Verification items for the finished model (mm, model axes). Face numbers are marked on the shaded views. A direction names the side the tool comes from. Give positions to 0.01 mm unless a question says otherwise; leave off trailing zeros. Write each loop counter-clockwise with the first axis right and the second up, starting at its lowest first coordinate (ties: lowest second). Pieces come first, ordered by that corner, then holes. Notation, with made-up numbers: M 65.25,40.25 L 100.25,40.25 A12 cw 100.25,45.25 Z; hole C 50,12.25 d3. An arc over 180 degrees is marked long. Answer as a JSON object with one key per item and string values.
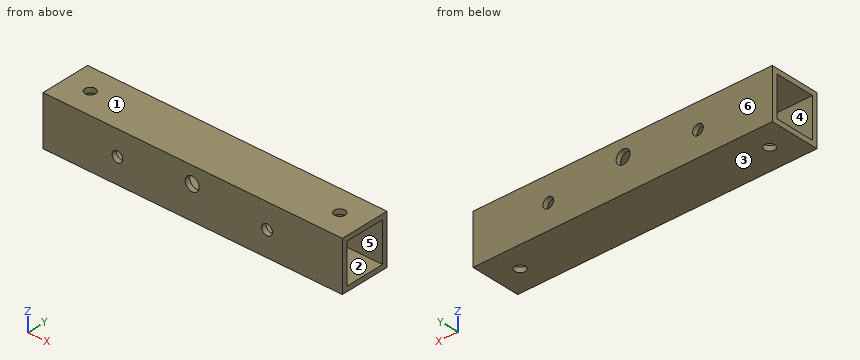
```python
from build123d import *

# Parameters (mm, degrees)
SKETCH_1_W          = 15
SKETCH_1_H          = 15
SKETCH_1_W_2        = 12
SKETCH_1_H_2        = 12
EXTRUDE_1_DEPTH     = 90
SKETCH_2_R          = 2.1
SKETCH_2_R_2        = 1.6
CUT_EXTRUDE_1_DEPTH = 92.549167118
SKETCH_3_R          = 1.6
CUT_EXTRUDE_2_DEPTH = 92.549167118


with BuildPart() as part:
    # ｽｹｯﾁ1 → ﾎﾞｽ - 押し出し1 (new body)
    with BuildSketch(Plane(origin=(0, 0, 0), x_dir=(0, 0, -1), z_dir=(1, 0, 0))):
        Rectangle(SKETCH_1_W, SKETCH_1_H)
        Rectangle(SKETCH_1_W_2, SKETCH_1_H_2, mode=Mode.SUBTRACT)
    extrude(amount=EXTRUDE_1_DEPTH)

    # ｽｹｯﾁ2 → ｶｯﾄ - 押し出し1 (cut, through all)
    with BuildSketch(Plane(origin=(0, 7.5, 0), x_dir=(1, 0, 0), z_dir=(0, 1, 0))):
        with Locations(Location((44.860461956, -2.501947466, 0), (0, 0, 270))):
            Circle(SKETCH_2_R)
        with Locations(Location((22.360461956, 0, 0), (0, 0, 270))):
            Circle(SKETCH_2_R_2)
        with Locations(Location((67.360461956, 0, 0), (0, 0, 270))):
            Circle(SKETCH_2_R_2)
    extrude(amount=-CUT_EXTRUDE_1_DEPTH, mode=Mode.SUBTRACT)

    # ｽｹｯﾁ3 → ｶｯﾄ - 押し出し2 (cut, through all)
    with BuildSketch(Plane.XY.offset(7.5)):
        with Locations((7.5, 0)):
            Circle(SKETCH_3_R)
        with Locations((82.5, 0)):
            Circle(SKETCH_3_R)
    extrude(amount=-CUT_EXTRUDE_2_DEPTH, mode=Mode.SUBTRACT)


solid = part.part
```
1) Section check C-C on x = 82.5. Record the boundary of the cut face in (y, z).
Completed:
{"outline": "M -7.5,-7.5 L -1.6,-7.5 L -1.6,-6 L -6,-6 L -6,6 L -1.6,6 L -1.6,7.5 L -7.5,7.5 Z; M 1.6,-7.5 L 7.5,-7.5 L 7.5,7.5 L 1.6,7.5 L 1.6,6 L 6,6 L 6,-6 L 1.6,-6 Z"}
2) Section check A-A on z = -4.5. Record the boundary of the cut face in (x, y), and give its area (3 significant figures).
Completed:
{"outline": "M 0,-7.5 L 90,-7.5 L 90,-6 L 0,-6 Z; M 0,6 L 90,6 L 90,7.5 L 0,7.5 Z", "area": "270 mm2"}
3) Section check D-D on x = 70. Record the boundary of the cut face in (y, z).
Completed:
{"outline": "M -7.5,-7.5 L 7.5,-7.5 L 7.5,7.5 L -7.5,7.5 Z; hole M -6,-6 L 6,-6 L 6,6 L -6,6 Z"}
4) Go/stop test with a flat-tipped pin: pin 1 (1 mm diameter, centred on y = -4, z = -5, fed in from -X). Record where the tip stops, or that it passes through.
Completed:
{"pin 1": "passes through"}
5) Release check for a two-part mould opening along Z. For the marked faces 3, 4, 5 and 6 record: pulls with the +Z half, pulls with the -Z half, needs draft (parallel to the pull), parting line crosses it, or undercut.
Completed:
{"face 3": "pulls with the -Z half", "face 4": "undercut", "face 5": "undercut", "face 6": "needs draft"}
6) Thickness scan on L1, parallel to Z at x = 11.5, y = 5; L2, parallel to Z at x = 67.5, y = -6.75. Record the ranges inside material, lowest first.
Completed:
{"L1": "z = -7.5 to -6, 6 to 7.5", "L2": "z = -7.5 to -1.59, 1.59 to 7.5"}
7) Access from +Z, -Z, +X, -X, +Y, -Y to the whole of each face (thin tool, end or side, straight path). Record for the marked faces 1 and 2.
Completed:
{"face 1": "+Z, +X, -X, +Y, -Y", "face 2": "+X, -X"}
